Here's the drawing with two shaded views (mm, measured from the low corner). I have some questions. A direction names the side the tool comes from. Round coordinates to 2 decimals unless told otherwise and drop trailing zeros. Order: outer loops, then holes, each group sorted by start corner. A loop starts at its lowest first (then second) coordinate and runs counter-clockwise, first axis right, second up. Notation, with made-up numbers: M -9.75,-7.75 L 45.25,-7.75 A12 cw 45.25,6.25 Z; hole C 53.5,7 d1. An arc over 180 degrees is marked long. One line per question, with ' | ' between items.
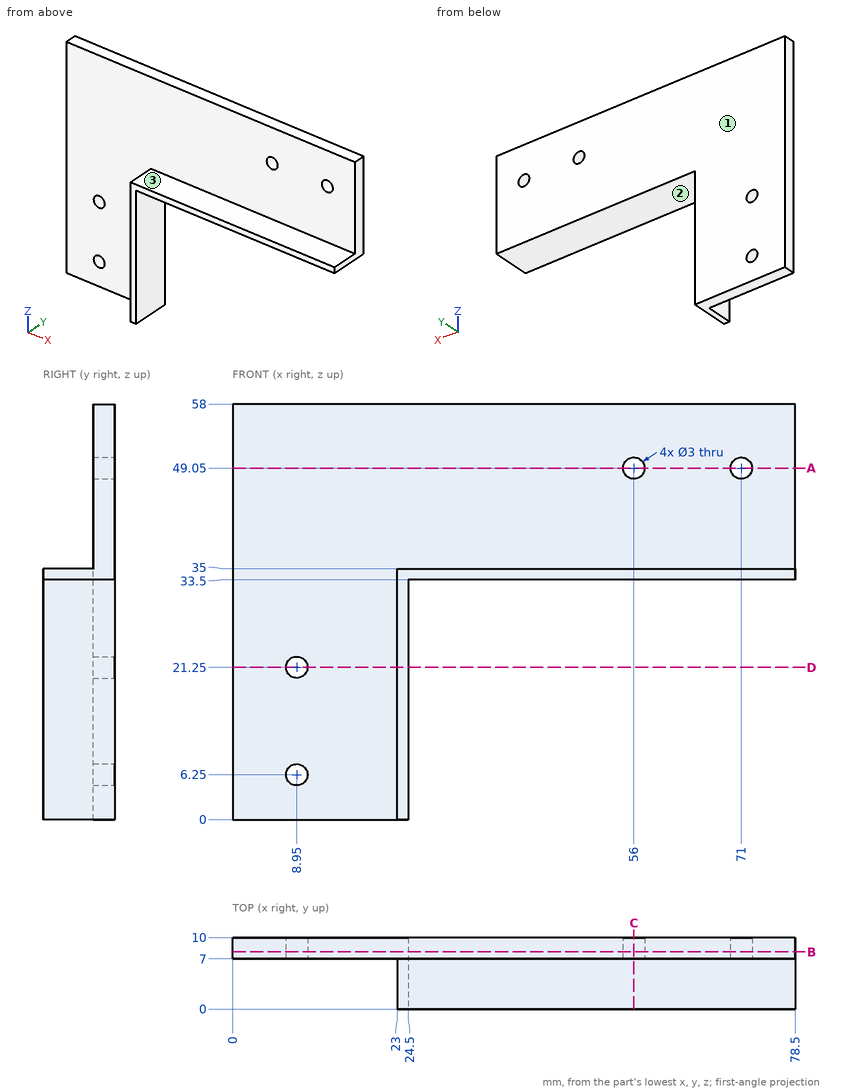
(1) If we section it at B-B on y = 8: Please give me the cut outline in (x, z), plus the area to 3 significant figures.
Final values:
outline: M 0,0 L 24.5,0 L 24.5,33.5 L 78.5,33.5 L 78.5,58 L 0,58 Z; hole C 8.95,6.25 d3; hole C 8.95,21.25 d3; hole C 56,49.05 d3; hole C 71,49.05 d3 | area: 2,720 mm^2
(2) If we section it at A-A on z = 49.05: Please give me the cut outline in (x, y).
Final values:
outline: M 0,7 L 54.5,7 L 54.5,10 L 0,10 Z; M 57.5,7 L 69.5,7 L 69.5,10 L 57.5,10 Z; M 72.5,7 L 78.5,7 L 78.5,10 L 72.5,10 Z
(3) On a 3-axis mill with a long thin cutter (end or side, diameter ignored), from which of +Z, -Z, +X, -X, +Y, -Y can I reach the whole of each face in a straight line? I mean the marked faces 1, 2 and 3. Say none if no direction works.
Final values:
face 1: +Z, -Z, +X, -X, +Y | face 2: -Z, +X, +Y, -Y | face 3: +Z, +X, -X, -Y
(4) Will these pins go through, and if not, where does the flat tip stop? pin 1 Ø1 at (y, z) = (4.5, 31.5) entering from +X; pin 2 Ø3.5 at (x, z) = (8.95, 6.25) entering from -Y; pin 3 Ø2.5 at (x, z) = (8.95, 21.25) entering from +Y; pin 4 Ø2 at (x, y) = (27.5, 2) entering from -Z.
Final values:
pin 1: x = 24.5 | pin 2: y = 7 | pin 3: through | pin 4: z = 33.5
(5) Please list where these lines run through material, in increasing order: probe 1 along X at (y, z) = (8.7, 49.05); probe 2 along X at (y, z) = (7.65, 21.25); probe 3 along Z at (x, y) = (8.95, 7.9). Write a range as [from, to].
Final values:
probe 1: [0, 54.5], [57.5, 69.5], [72.5, 78.5] | probe 2: [0, 7.45], [10.45, 24.5] | probe 3: [0, 4.75], [7.75, 19.75], [22.75, 58]
(6) If we section it at D-D on z = 21.25: Please give me the cut outline in (x, y), plus the area to 3 significant figures.
Final values:
outline: M 0,7 L 7.45,7 L 7.45,10 L 0,10 Z; M 10.45,7 L 23,7 L 23,0 L 24.5,0 L 24.5,10 L 10.45,10 Z | area: 75.0 mm^2
(7) If we section it at C-C on x = 56: Please give me the cut outline in (y, z), plus the area to 3 significant figures.
Final values:
outline: M 0,33.5 L 10,33.5 L 10,47.55 L 7,47.55 L 7,35 L 0,35 Z; M 7,50.55 L 10,50.55 L 10,58 L 7,58 Z | area: 75.0 mm^2
